The listing builds one solid part. Answer for the finished solid, in the listing's coordinates (mm). A direction names the side the tool comes from. Round coordinates to 2 decimals unless told otherwise and drop trailing zeros. Write each loop counter-clockwise with the first axis right and the second up, starting at its lowest first coordinate (ties: lowest second). Pieces come first, ordered by that corner, then holes.
from build123d import *

# Parameters (mm, degrees)
EXTRUDE1_DEPTH      = 22.61
CHAMFER1_SIZE       = 2.54
SKETCH2_R           = 0.76
CUT_EXTRUDE1_DEPTH  = 31.446849151
EXTRUDE2_DEPTH      = 31.446849151
EXTRUDE2_DEPTH_BACK = 31.446849151
SKETCH3_W           = 6.352
SKETCH3_H           = 3.664879672


with BuildPart() as part:
    # Sketch1 → Extrude1 (new body)
    with BuildSketch(Plane.XY):
        with BuildLine():
            Line((-1.27, 20.32), (-1.701415211, 0.036187299))
            ThreePointArc((-1.701415211, 0.036187299), (0, -1.7018), (1.701415211, 0.036187299))
            Line((1.701415211, 0.036187299), (1.27, 20.32))
            Line((1.27, 20.32), (-1.27, 20.32))
        make_face()
    extrude(amount=-EXTRUDE1_DEPTH)

    # Chamfer1
    chamfer1_edges = [part.edges().sort_by_distance(p)[0] for p in [
        (0, 20.32, -22.61),
        (0, 20.32, 0),
    ]]
    chamfer(chamfer1_edges, length=CHAMFER1_SIZE)

    # Sketch2 → Cut-Extrude1 (cut, through all)
    with BuildSketch(Plane.XY):
        Circle(SKETCH2_R)
    extrude(amount=-CUT_EXTRUDE1_DEPTH, mode=Mode.SUBTRACT)

    # Sketch3 → Extrude2 (cut, two sides: drawn at the far end of the back side and taken through both)
    with BuildSketch(Plane(origin=(0, 0, 0), x_dir=(0, 0, -1), z_dir=(1, 0, 0)).offset(-EXTRUDE2_DEPTH_BACK)):
        with Locations((3.176, 0.130639836)):
            Rectangle(SKETCH3_W, SKETCH3_H)
        with Locations((19.434, 0.130639836)):
            Rectangle(SKETCH3_W, SKETCH3_H)
    extrude(amount=EXTRUDE2_DEPTH + EXTRUDE2_DEPTH_BACK, mode=Mode.SUBTRACT)


solid = part.part
1. Section A-A on x = 0 is taken. Determine the outline of the cut face in (y, z), plus the area to 3 significant figures.
Geometry says:
outline: (-1.7, -16.26) - (-0.76, -16.26) - (-0.76, -6.35) - (-1.7, -6.35) - close; (0.76, -16.26) - (1.96, -16.26) - (1.96, -22.61) - (17.78, -22.61) - (20.32, -20.07) - (20.32, -2.54) - (17.78, 0) - (1.96, 0) - (1.96, -6.35) - (0.76, -6.35) - close
area: 430 mm2
2. Section D-D on y = 5 is taken. Determine the outline of the cut face in (x, z).
Geometry says:
outline: (-1.6, -22.61) - (1.6, -22.61) - (1.6, 0) - (-1.6, 0) - close
3. Section B-B on z = -8.25 is taken. Determine the outline of the cut face in (x, y), plus the area to 3 significant figures.
Geometry says:
outline: (-1.7, 0.04) arc R1.7 ccw (long way) to (1.7, 0.04) - (1.27, 20.32) - (-1.27, 20.32) - close; hole circle Ø1.52 at (0, 0)
area: 63.1 mm2
4. Section C-C on z = -3.25 is taken. Determine the outline of the cut face in (x, y).
Geometry says:
outline: (-1.66, 1.96) - (1.66, 1.96) - (1.27, 20.32) - (-1.27, 20.32) - close
5. Straight lines are drawn through the part: line 1 along Y through (x, z) = (0, -9.75); line 2 along Z through (x, y) = (1.35, -0.25); line 3 along Y through (x, z) = (-0.35, -15). For each, find the intervals that lie inside material, in ascending order.
Geometry says:
line 1: y = -1.7 to -0.76, 0.76 to 20.32
line 2: z = -16.26 to -6.35
line 3: y = -1.67 to -0.67, 0.67 to 20.32
6. For a pull along X with two mould halves and no side action, classify faces 1 (the face through (0, -1.7, -11.2)), 2 (the face through (0.725, 0.228, -11.236)), 3 (the face through (0, 1, -16.258)) as released by +X, released by -X, zero draft, split by the parting line, or undercut.
Geometry says:
face 1: split by the parting line
face 2: undercut
face 3: zero draft
7. A tool of negligible diameter and unlimited length cuts with its end or side. For faces 4 (the face through (0, 1, -6.352)), 5 (the face through (0, 1.963, -19)), 6 (the face through (0, 10, -22.61)), from which of +Z, -Z, +X, -X, +Y, -Y can it reach the whole face along a straight path? Write none if from no direction.
Geometry says:
face 4: +Z, +X, -X, -Y
face 5: -Z, +X, -X, -Y
face 6: -Z, +X, -X, +Y, -Y
8. Given pin 1 (6 mm diameter, centred on y = 5.5, z = -4, fed in from -X); pin 2 (4 mm diameter, centred on y = 4, z = -20.5, fed in from +X); pin 3 (1.4 mm diameter, centred on x = 0, y = 0, fed in from -Z); pin 4 (2 mm diameter, centred on y = 15, z = -6, fed in from +X), each flat-ended and moving along its own axis, determine where each tip first touches the part or whether it passes through.
Geometry says:
pin 1: stops at x = -1.65
pin 2: stops at x = 1.66
pin 3: passes through
pin 4: stops at x = 1.4
